Build history of the part. All positions in model axes, mm. Face numbers are marked on the shaded views. A direction names the side the tool comes from. Give positions to 0.01 mm unless a question says otherwise; leave off trailing zeros. Loops run counter-clockwise (first coordinate to the right, second up) from the corner with the lowest first, then second, coordinate; pieces in that order, holes last. Notation, with made-up numbers: M 9,-39 L 34,-39 A6 ccw 34,-33 Z; hole C 24,-10.75 d8. An arc over 180 degrees is marked long. Answer as a JSON object with one key per item and string values. Group by question number.
1. Slice it at A-A (y = -27.7). List the corners of the cut face in (x, z).
2. Drop flat-ended pins along their axis: pin 1 Ø1 at (y, z) = (-6.5, -17) entering from -X; pin 2 Ø6.5 at (y, z) = (-28, -9.5) entering from +X. Give the stop position or say it passes through.
3. Slice it at B-B (z = -23.75). List the corners of the cut face in (x, y).
4. 3-axis set-ups, long thin cutter, end or side, ignore diameter. For the marked faces 1, 2 and 3: which of +Z, -Z, +X, -X, +Y, -Y reach the whole face in a straight line?
5. Drill centre lines: line 1 along Z through (x, y) = (1.85, -27.7); line 2 along Z through (x, y) = (2.5, -28.75); line 3 along Y through (x, z) = (2.5, -4.5). Where is each one in solid material? Low to high. Write a range as [from, to].
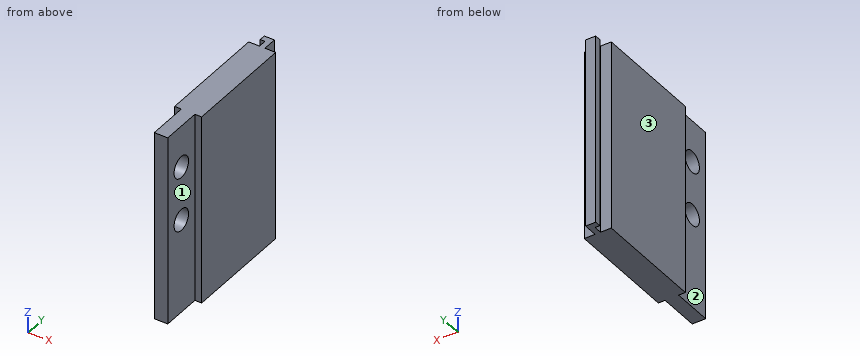
from build123d import *

# Parameters (mm, degrees)
SKETCH_1_W          = 0.8
SKETCH_1_H          = 2.1
SKETCH_1_W_2        = 2
SKETCH_1_H_2        = 6
SKETCH_1_W_3        = 0.7
SKETCH_1_H_3        = 0.9
EXTRUDE_1_DEPTH     = 20
SKETCH_3_R          = 1.6
CUT_EXTRUDE_1_DEPTH = 37.762616882
EXTRUDE_2_DEPTH     = 8.208511786


with BuildPart() as part:
    # 草图1 → 凸台-拉伸1 (new body)
    with BuildSketch(Plane.XY):
        with Locations((2, -7.25)):
            Rectangle(SKETCH_1_W, SKETCH_1_H)
        Polygon((4, -8.3), (2.4, -8.3), (1.6, -8.3), (0, -8.3), (0, -24.7), (1, -24.7), (3, -24.7), (4, -24.7), align=None)
        with Locations((2, -27.7)):
            Rectangle(SKETCH_1_W_2, SKETCH_1_H_2)
        with Locations((1.25, -6.65)):
            Rectangle(SKETCH_1_W_3, SKETCH_1_H_3)
    extrude(amount=-EXTRUDE_1_DEPTH)

    # 草图3 → 切除-拉伸1 (cut, through all)
    with BuildSketch(Plane(origin=(3, 0, 0), x_dir=(0, 0, -1), z_dir=(1, 0, 0))):
        with Locations(Location((6.208511786, -27.7, 0), (0, 0, 90))):
            Circle(SKETCH_3_R)
        with Locations(Location((14.208511786, -27.7, 0), (0, 0, 90))):
            Circle(SKETCH_3_R)
    extrude(amount=-CUT_EXTRUDE_1_DEPTH, mode=Mode.SUBTRACT)

    # 草图4 → 凸台-拉伸2 (add)
    with BuildSketch(Plane(origin=(0, 0, -20), x_dir=(-1, 0, 0), z_dir=(0, 0, -1))):
        Polygon((-0.9, -6.2), (-2.4, -6.2), (-2.4, -8.3), (-4, -8.3), (-4, -24.7), (-3, -24.7), (-3, -30.7), (-1, -30.7), (-1, -24.7), (0, -24.7), (0, -8.3), (-1.6, -8.3), (-1.6, -7.1), (-0.9, -7.1), align=None)
    extrude(amount=EXTRUDE_2_DEPTH)


solid = part.part
Established:
{
 "1": {"outline": "M 1,-28.21 L 3,-28.21 L 3,-15.81 L 1,-15.81 Z; M 1,-12.61 L 3,-12.61 L 3,-7.81 L 1,-7.81 Z; M 1,-4.61 L 3,-4.61 L 3,0 L 1,0 Z"},
 "2": {"pin 1": "stops at x = 0.9", "pin 2": "stops at x = 3"},
 "3": {"outline": "M 0,-24.7 L 1,-24.7 L 1,-30.7 L 3,-30.7 L 3,-24.7 L 4,-24.7 L 4,-8.3 L 2.4,-8.3 L 2.4,-6.2 L 0.9,-6.2 L 0.9,-7.1 L 1.6,-7.1 L 1.6,-8.3 L 0,-8.3 Z"},
 "4": {"face 1": "+Z, -Z, +X, -Y", "face 2": "+Z, -Z, -X, -Y", "face 3": "+Z, -Z, -X, +Y, -Y"},
 "5": {"line 1": "z = [-28.21, -15.81], [-12.61, -7.81], [-4.61, 0]", "line 2": "z = [-28.21, -15.42], [-13, -7.42], [-5, 0]", "line 3": "y = [-30.7, -8.3]"}
}
